```python
from build123d import *

# Parameters (mm, degrees)
SKETCH1_R           = 3.8
SKETCH1_R_2         = 1.65
BOSS_EXTRUDE1_DEPTH = 20.4
CHAMFER1_SIZE       = 4
CHAMFER1_SIZE2      = 0.850226247
CHAMFER2_SIZE       = 4
CHAMFER2_SIZE2      = 0.850226247


with BuildPart() as part:
    # Sketch1 → Boss-Extrude1 (new body)
    with BuildSketch(Plane.XY):
        Circle(SKETCH1_R)
        Circle(SKETCH1_R_2, mode=Mode.SUBTRACT)
    extrude(amount=BOSS_EXTRUDE1_DEPTH)

    # Chamfer1
    chamfer1_edges = [part.edges().sort_by_distance(p)[0] for p in [
        (-3.8, 0, 20.4),
    ]]
    chamfer1_side = [part.faces().sort_by_distance(p)[0] for p in [
        (-3.8, 0, 10.2),
    ]]
    chamfer(chamfer1_edges, length=CHAMFER1_SIZE, length2=CHAMFER1_SIZE2, reference=chamfer1_side[0])

    # Chamfer2
    chamfer2_edges = [part.edges().sort_by_distance(p)[0] for p in [
        (-3.8, 0, 0),
    ]]
    chamfer2_side = [part.faces().sort_by_distance(p)[0] for p in [
        (-3.8, 0, 8.2),
    ]]
    chamfer(chamfer2_edges, length=CHAMFER2_SIZE, length2=CHAMFER2_SIZE2, reference=chamfer2_side[0])


solid = part.part
```
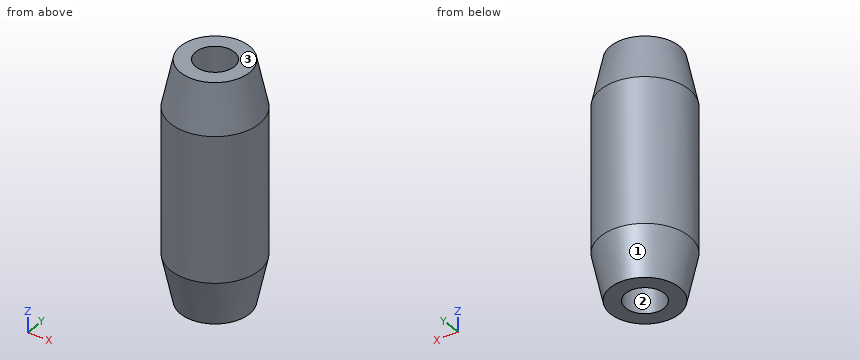
Model file for the job. Use its own axes, mm. Face numbers are marked on the shaded views. Give positions to 0.01 mm unless a question says otherwise; leave off trailing zeros. Order: outer loops, then holes, each group sorted by start corner. A loop starts at its lowest first (then second) coordinate and runs counter-clockwise, first axis right, second up.
1) Wall check: probe 1 along Y at (x, z) = (0, 5); probe 2 along X at (y, z) = (-1, 2); probe 3 along Y at (x, z) = (-2.5, 8). Give the ranges that are in metal, low to high.
2) Mould opens along Y. For the marked faces 1, 2 and 3 say: +Y half, -Y half, draft (parallel to the pull), parting line (faces both ways), or undercut.
3) Saw through at C-C, the plane z = 14.75. Write the cut outline in (x, y), then the cut area to 3 significant figures.
4) Pin check, flat tip, straight feed: pin 1 (1 mm diameter, centred on y = -3, z = 3.5, fed in from +X). Stop position of the tip, or through.
5) Saw through at A-A, the plane x = 0. Write the cut outline in (y, z).
Computed:
1. probe 1: y = -3.8 to -1.65, 1.65 to 3.8
1. probe 2: x = -3.22 to -1.31, 1.31 to 3.22
1. probe 3: y = -2.86 to 2.86
2. face 1: parting line
2. face 2: undercut
2. face 3: draft
3. outline: circle Ø7.6 at (0, 0); hole circle Ø3.3 at (0, 0)
3. area: 36.8 mm2
4. pin 1: stops at x = 2.74
5. outline: (-3.8, 4) - (-2.95, 0) - (-1.65, 0) - (-1.65, 20.4) - (-2.95, 20.4) - (-3.8, 16.4) - close; (1.65, 0) - (2.95, 0) - (3.8, 4) - (3.8, 16.4) - (2.95, 20.4) - (1.65, 20.4) - close
